from build123d import *

# Parameters (mm, degrees)
SKETCH1_W           = 29.845
SKETCH1_H           = 24.003
SKETCH1_R           = 5.83565
BOSS_EXTRUDE1_DEPTH = 1.9812
SKETCH7_W           = 24.003
SKETCH7_H           = 31.8262
BOSS_EXTRUDE4_DEPTH = 1.9812
BOSS_EXTRUDE5_DEPTH = 1.9812
BOSS_EXTRUDE6_DEPTH = 1.9812
SKETCH10_W          = 6.4
SKETCH10_H          = 31.8262
BOSS_EXTRUDE7_DEPTH = 23.2664
SKETCH11_R          = 2.349999999
CUT_EXTRUDE1_DEPTH  = 65.474833866


with BuildPart() as part:
    # Sketch1 → Boss-Extrude1 (new body)
    with BuildSketch(Plane(origin=(0, 0, 0), x_dir=(1, 0, 0), z_dir=(0, 1, 0))):
        with Locations((-14.9225, 12.0015)):
            Rectangle(SKETCH1_W, SKETCH1_H)
        with Locations(Location((-14.9225, 12.0015, 0), (0, 0, 270))):
            Circle(SKETCH1_R, mode=Mode.SUBTRACT)
    extrude(amount=BOSS_EXTRUDE1_DEPTH)

    # Sketch7 → Boss-Extrude4 (add)
    with BuildSketch(Plane.ZY.offset(29.845)):
        with Locations((-12.0015, -13.9319)):
            Rectangle(SKETCH7_W, SKETCH7_H)
    extrude(amount=BOSS_EXTRUDE4_DEPTH)

    # Sketch8 → Boss-Extrude5 (add)
    with BuildSketch(Plane.XY):
        Polygon((-29.845, -29.845), (-29.845, 0), (0, 0), align=None)
    extrude(amount=-BOSS_EXTRUDE5_DEPTH)

    # Sketch9 → Boss-Extrude6 (add)
    with BuildSketch(Plane(origin=(0, 0, -24.003), x_dir=(-1, 0, 0), z_dir=(0, 0, -1))):
        Polygon((0, 0), (29.845, 0), (29.845, -29.845), align=None)
    extrude(amount=-BOSS_EXTRUDE6_DEPTH)

    # Sketch10 → Boss-Extrude7 (add)
    with BuildSketch(Plane.ZY.offset(31.8262)):
        with Locations((-12.0015, -13.9319)):
            Rectangle(SKETCH10_W, SKETCH10_H)
    extrude(amount=BOSS_EXTRUDE7_DEPTH)

    # Sketch11 → Cut-Extrude1 (cut, through all)
    with BuildSketch(Plane.XY.offset(-8.8015)):
        with Locations((-50.710600001, -25.908)):
            Circle(SKETCH11_R)
        with Locations((-36.260599945, -25.908)):
            Circle(SKETCH11_R)
    extrude(amount=-CUT_EXTRUDE1_DEPTH, mode=Mode.SUBTRACT)


solid = part.part
Verification items for the finished model (mm, model axes). A direction names the side the tool comes from. Coordinates: 2 decimals unless noted, no trailing zeros. Loops run counter-clockwise (first coordinate to the right, second up) from the corner with the lowest first, then second, coordinate; pieces in that order, holes last. Notation, with made-up numbers: (79, 3.5) -> (105, 3.5) arc R20 ccw to (105, 36.5) -> close; hole circle Ø6 at (60.5, 1.25). An arc over 180 degrees is marked (long way). Write each question's results on one line, items separated by ' | '.
Item 1: Gauge pin test, flat ends, axial feed: pin 1 (6 mm diameter, centred on x = -14.5, z = -14, fed in from -Y); pin 2 (18.5 mm diameter, centred on x = -42, y = -21.5, fed in from -Z); pin 3 (8 mm diameter, centred on y = -12, z = -15, fed in from +X) (3 decimals); pin 4 (7.5 mm diameter, centred on x = -36.26, y = -25.91, fed in from +Z). Record the tip position at first contact, or that the pin passes through.
Found:
pin 1: passes through | pin 2: stops at z = -15.2 | pin 3: stops at x = -29.845 | pin 4: stops at z = -8.8
Item 2: Tool access check on faces 1 (the face through (-43, -14, -8.802)), 2 (the face through (-20, -10, -24.003)), 3 (the face through (-43, -14, -15.202)), 4 (the face through (-18, -11, -22.022)). Record the directions out of +Z, -Z, +X, -X, +Y, -Y that give a thin tool (end or side, any length) a straight path to the whole face; none if there is none.
Found:
face 1: +Z, -X, +Y, -Y | face 2: -Z, +X, -X, +Y, -Y | face 3: -Z, -X, +Y, -Y | face 4: +X, -Y
Item 3: Section check B-B, the plane x = -35.5. Enter the section's corners in (y, z) (1 decimal).
Found:
outline: (-29.8, -15.2) -> (-28.1, -15.2) -> (-28.1, -8.8) -> (-29.8, -8.8) -> close; (-23.7, -15.2) -> (2, -15.2) -> (2, -8.8) -> (-23.7, -8.8) -> close
Item 4: Material ranges on L1, parallel to Z at x = -25, y = -15; L2, parallel to X at y = -26.5, z = -9.25 (3 decimals); L3, parallel to X at y = -0.5, z = -13.25 (3 decimals), recorded low to high.
Found:
L1: z = -24 to -22.02, -1.98 to 0 | L2: x = -55.093 to -52.985, -48.436 to -38.535, -33.986 to -29.845 | L3: x = -55.093 to -29.845
Item 5: Section check D-D, the plane z = -10.25. Enter the section's corners in (x, y) (3 decimals).
Found:
outline: (-55.093, -29.845) -> (-29.845, -29.845) -> (-29.845, 0) -> (-20.489, 0) -> (-20.489, 1.981) -> (-55.093, 1.981) -> close; (-9.356, 0) -> (0, 0) -> (0, 1.981) -> (-9.356, 1.981) -> close; hole circle Ø4.7 at (-50.711, -25.908); hole circle Ø4.7 at (-36.261, -25.908)
Item 6: Section check A-A, the plane z = -6.75. Enter the section's corners in (x, y) (3 decimals), plus the area to 3 significant figures.
Found:
outline: (-31.826, -29.845) -> (-29.845, -29.845) -> (-29.845, 0) -> (-17.467, 0) -> (-17.467, 1.981) -> (-31.826, 1.981) -> close; (-12.378, 0) -> (0, 0) -> (0, 1.981) -> (-12.378, 1.981) -> close | area: 112 mm2
Item 7: Section check C-C, the plane y = -27. Enter the section's corners in (x, z) (1 decimal).
Found:
outline: (-55.1, -15.2) -> (-52.8, -15.2) -> (-52.8, -8.8) -> (-55.1, -8.8) -> close; (-48.6, -15.2) -> (-38.3, -15.2) -> (-38.3, -8.8) -> (-48.6, -8.8) -> close; (-34.2, -15.2) -> (-31.8, -15.2) -> (-31.8, -24) -> (-27, -24) -> (-27, -22) -> (-29.8, -22) -> (-29.8, -2) -> (-27, -2) -> (-27, 0) -> (-31.8, 0) -> (-31.8, -8.8) -> (-34.2, -8.8) -> close
Item 8: Mould release check, pull along X, two halves, no side actions. Record for faces 5 (the face through (-31.826, -14, -20)), 6 (the face through (-19, -10, 0)), 7 (the face through (-10.978, 0.977, -16.303)): +X half, -X half, draft (parallel to the pull), parting line (faces both ways), or undercut.
Found:
face 5: -X half | face 6: draft | face 7: undercut
